```python
from build123d import *

# Parameters (mm, degrees)
SKETCH1_W             = 22
SKETCH1_H             = 55
BASE_DEPTH            = 5
SKETCH2_R             = 12
MOTOR_SUPPORT_DEPTH   = 22
SKETCH3_W             = 8
SKETCH3_H             = 8
CLAMP_FLANGE_DEPTH    = 22
SKETCH4_W             = 2.208433096
SKETCH4_H             = 15
SLOT_DEPTH            = 35
F_6_CLEARANCE_HOLE1_D = 3.7973
HEX_CUT_DEPTH         = 56.463952257
HEX_CUT_DEPTH_BACK    = 1.5
SKETCH9_R             = 3.5
SCREW_HEAD_CUT_DEPTH  = 56.463952257
MOUNTING_SLOT_DEPTH   = 50.651284016
LPATTERN1_COUNT       = 2
LPATTERN1_PITCH       = 12
LPATTERN1_COUNT_DIR2  = 2
LPATTERN1_PITCH_DIR2  = 43
FILLET2_R             = 5
FILLET3_R             = 1
FILLET4_R             = 10


with BuildPart() as part:
    # Sketch1 → Base (new body)
    with BuildSketch(Plane(origin=(0, 0, 0), x_dir=(1, 0, 0), z_dir=(0, 1, 0))):
        with Locations((-11, 0)):
            Rectangle(SKETCH1_W, SKETCH1_H)
    extrude(amount=BASE_DEPTH)

    # Sketch2 → Motor Support (add)
    with BuildSketch(Plane(origin=(0, 0, 0), x_dir=(0, 0, -1), z_dir=(1, 0, 0))):
        with BuildLine():
            Line((-14, 20), (-14, 0))
            Line((-14, 0), (14, 0))
            Line((14, 0), (14, 20))
            ThreePointArc((14, 20), (0, 34), (-14, 20))
        make_face()
        with Locations((0, 20)):
            Circle(SKETCH2_R, mode=Mode.SUBTRACT)
    extrude(amount=-MOTOR_SUPPORT_DEPTH)

    # Sketch3 → Clamp Flange (add)
    with BuildSketch(Plane(origin=(0, 0, 0), x_dir=(0, 0, -1), z_dir=(1, 0, 0))):
        with Locations((0, 36)):
            Rectangle(SKETCH3_W, SKETCH3_H)
    extrude(amount=-CLAMP_FLANGE_DEPTH)

    # Sketch4 → Slot (cut)
    with BuildSketch(Plane(origin=(0, 0, 0), x_dir=(0, 0, -1), z_dir=(1, 0, 0))):
        with Locations((0, 33.5)):
            Rectangle(SKETCH4_W, SKETCH4_H)
    extrude(amount=-SLOT_DEPTH, mode=Mode.SUBTRACT)

    # #6 Clearance Hole1 (through all)
    with Locations(Plane.XY.offset(4)):
        with Locations((-11, 36)):
            Hole(F_6_CLEARANCE_HOLE1_D / 2)

    # Sketch7 → Hex-Cut (cut, two sides: drawn at the far end of the back side and taken through both)
    with BuildSketch(Plane.XY.offset(4).offset(-HEX_CUT_DEPTH_BACK)):
        Polygon((-8.690598923, 40), (-13.309401077, 40), (-15.618802154, 36), (-13.309401077, 32), (-8.690598923, 32), (-6.381197846, 36), align=None)
    extrude(amount=HEX_CUT_DEPTH + HEX_CUT_DEPTH_BACK, mode=Mode.SUBTRACT)

    # Sketch9 → Screw Head Cut (cut, through all)
    with BuildSketch(Plane(origin=(0, 0, -4), x_dir=(-1, 0, 0), z_dir=(0, 0, -1))):
        with Locations((11, 36)):
            Circle(SKETCH9_R)
    extrude(amount=SCREW_HEAD_CUT_DEPTH, mode=Mode.SUBTRACT)

    # Sketch8 → Mounting Slot (cut, through all)
    with BuildSketch(Plane(origin=(0, 5, 0), x_dir=(1, 0, 0), z_dir=(0, 1, 0))):
        with BuildLine():
            Line((-18.75, 19.5), (-18.75, 24.5))
            ThreePointArc((-18.75, 24.5), (-17, 26.25), (-15.25, 24.5))
            Line((-15.25, 24.5), (-15.25, 19.5))
            ThreePointArc((-15.25, 19.5), (-17, 17.75), (-18.75, 19.5))
        make_face()
    mounting_slot = extrude(amount=-MOUNTING_SLOT_DEPTH, mode=Mode.SUBTRACT)

    # LPattern1: Mounting Slot 2 × 2
    with Locations(*[(i * LPATTERN1_PITCH, 0, j * LPATTERN1_PITCH_DIR2) for i in range(LPATTERN1_COUNT) for j in range(LPATTERN1_COUNT_DIR2) if (i, j) != (0, 0)]):
        add(mounting_slot, mode=Mode.SUBTRACT)

    # Fillet2
    fillet2_edges = [part.edges().sort_by_distance(p)[0] for p in [
        (0, 2.5, 27.5),
        (-22, 2.5, 27.5),
        (-22, 2.5, -27.5),
        (0, 2.5, -27.5),
    ]]
    fillet(fillet2_edges, radius=FILLET2_R)

    # Fillet3
    fillet3_edges = [part.edges().sort_by_distance(p)[0] for p in [
        (-11, 5, -14),
        (-11, 5, 14),
    ]]
    fillet(fillet3_edges, radius=FILLET3_R)

    # Fillet4
    # the kernel refuses this fillet: 10 mm, written as the material it takes off along each edge
    with BuildSketch(Plane(origin=(0, 40, -29), x_dir=(0, -1, 0), z_dir=(0, 0, 1)), Plane(origin=(0, 40, -23.895783452), x_dir=(0, -1, 0), z_dir=(0, 0, 1))) as fillet4_piece_1:
        with BuildLine():
            CenterArc((FILLET4_R, -FILLET4_R), FILLET4_R, 90, 90)
            Line((0, -FILLET4_R), (0, 0))
            Line((0, 0), (FILLET4_R, 0))
        make_face()
    extrude(amount=52.895783452, mode=Mode.SUBTRACT)
    with BuildSketch(Plane(origin=(-22, 40, -29), x_dir=(0, -1, 0), z_dir=(0, 0, 1)), Plane(origin=(-22, 40, -23.895783452), x_dir=(0, -1, 0), z_dir=(0, 0, 1))) as fillet4_piece_2:
        with BuildLine():
            CenterArc((FILLET4_R, FILLET4_R), FILLET4_R, 180, 90)
            Line((0, FILLET4_R), (0, 0))
            Line((0, 0), (FILLET4_R, 0))
        make_face()
    extrude(amount=52.895783452, mode=Mode.SUBTRACT)


solid = part.part
```
CAD build for the part. Positions are in the model's coordinates, mm. A direction names the side the tool comes from. Give positions to 0.01 mm unless a question says otherwise; leave off trailing zeros. Loops run counter-clockwise (first coordinate to the right, second up) from the corner with the lowest first, then second, coordinate; pieces in that order, holes last. Notation, with made-up numbers: (-6, 41.25) - (25, 41.25) arc R20 cw to (25, 49.25) - close; hole circle Ø10 at (24.25, 8). An arc over 180 degrees is marked (long way). Put each result on its own line as item: value.
Q1. Slice it at A-A (y = 3.5). Give the cut face in (x, z), plus the area to 3 significant figures.
Filled in:
outline: (-22, -22.5) arc R5 ccw to (-17, -27.5) - (-5, -27.5) arc R5 ccw to (0, -22.5) - (0, 22.5) arc R5 ccw to (-5, 27.5) - (-17, 27.5) arc R5 ccw to (-22, 22.5) - close; hole (-18.75, -24.5) arc R1.75 ccw to (-15.25, -24.5) - (-15.25, -19.5) arc R1.75 ccw to (-18.75, -19.5) - close; hole (-18.75, 18.5) arc R1.75 ccw to (-15.25, 18.5) - (-15.25, 23.5) arc R1.75 ccw to (-18.75, 23.5) - close; hole (-6.75, -24.5) arc R1.75 ccw to (-3.25, -24.5) - (-3.25, -19.5) arc R1.75 ccw to (-6.75, -19.5) - close; hole (-6.75, 18.5) arc R1.75 ccw to (-3.25, 18.5) - (-3.25, 23.5) arc R1.75 ccw to (-6.75, 23.5) - close
area: 1,080 mm²
Q2. Slice it at C-C (y = 19). Give the cut face in (x, z), plus the area to 3 significant figures.
Filled in:
outline: (-22, -14) - (0, -14) - (0, -11.96) - (-22, -11.96) - close; (-22, 11.96) - (0, 11.96) - (0, 14) - (-22, 14) - close
area: 89.8 mm²
Q3. Slice it at D-D (z = -17). Give the cut face in (x, y), plus the area to 3 significant figures.
Filled in:
outline: (-22, 0) - (0, 0) - (0, 5) - (-22, 5) - close
area: 110 mm²
Q4. Mould opens along Y. For faces 4 (the face through (-5, 36, 4)), 5 (the face through (-11, 32.5, -4.9)), 6 (the face through (-7.493, 37.926, 3.24)), 7 (the face through (-10.85, 8.01, 0.51)) say: pulls with the +Y half, pulls with the -Y half, needs draft (parallel to the pull), parting line crosses it, or undercut.
Filled in:
face 4: needs draft
face 5: pulls with the +Y half
face 6: undercut
face 7: undercut
Q5. Probe line 1 along Z through (x, y) = (-15, 34); line 2 along X through (y, z) = (3.5, 22); line 3 along Y through (x, z) = (-11, -2.35). List the from-to ranges inside material, lowest first.
Filled in:
line 1: z = -4 to -1.1, 1.1 to 4
line 2: x = -22 to -18.75, -15.25 to -6.75, -3.25 to 0
line 3: y = 0 to 8.23, 31.77 to 34.1, 37.9 to 40
Q6. Slice it at B-B (x = -18). Give the cut face in (y, z).
Filled in:
outline: (0, -27.4) - (5, -27.4) - (5, -25.94) - (0, -25.94) - close; (0, -18.06) - (5, -18.06) - (5, -15) arc R1 cw to (6, -14) - (20, -14) arc R14 ccw to (33.42, -4) - (38, -4) - (38, -1.1) - (31.95, -1.1) arc R12 cw (long way) to (31.95, 1.1) - (38, 1.1) - (38, 4) - (33.42, 4) arc R14 ccw to (20, 14) - (6, 14) arc R1 cw to (5, 15) - (5, 17.06) - (0, 17.06) - close; (0, 24.94) - (5, 24.94) - (5, 27.4) - (0, 27.4) - close
Q7. Tool access for faces 1 (the face through (-11, 5, -21)), 2 (the face through (-3.25, 3, -22)), 3 (the face through (-11, 33, 1.104)): list every direction of +Z, -Z, +X, -X, +Y, -Y with a clear straight run to the whole face (end or side of a thin tool).
Filled in:
face 1: -Z, +X, -X, +Y
face 2: +Y, -Y
face 3: +X, -X, +Y
Q8. Flat gauge pins, fed straight in: pin 1 (2 mm diameter, centred on x = -18.5, z = -4.5, fed in from +Y); pin 2 (10 mm diameter, centred on x = -8.5, y = 28, fed in from +Z); pin 3 (1.9 mm diameter, centred on x = -17, y = 36, fed in from +Z); pin 4 (3 mm diameter, centred on x = -4.5, z = -4, fed in from -Y). Where does each tip first touch, or does it go through?
Filled in:
pin 1: stops at y = 38.26
pin 2: stops at z = 13.67
pin 3: stops at z = 4
pin 4: stops at y = 0
